Here's how the part is built. I have some questions about the finished solid (model axes, mm). Round coordinates to 2 decimals unless told otherwise and drop trailing zeros. Order: outer loops, then holes, each group sorted by start corner. A loop starts at its lowest first (then second) coordinate and runs counter-clockwise, first axis right, second up.
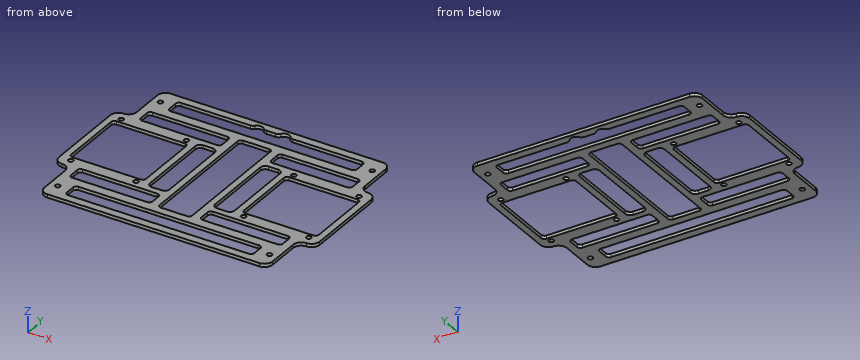
```python
from build123d import *

# Parameters (mm, degrees)
SKETCH_1_R          = 1.5
EXTRUDE_1_DEPTH     = 2
SKETCH_2_R          = 1.5
SKETCH_2_W          = 46
SKETCH_2_H          = 43
CUT_EXTRUDE_1_DEPTH = 2
FILLET_1_R          = 2
SKETCH_3_W          = 115
SKETCH_3_H          = 10
CUT_EXTRUDE_2_DEPTH = 2
FILLET_2_R          = 2
SKETCH_4_W          = 20
SKETCH_4_H          = 80
SKETCH_4_W_2        = 50
SKETCH_4_H_2        = 10
CUT_EXTRUDE_3_DEPTH = 2
FILLET_3_R          = 2
FILLET_4_R          = 5
SKETCH_5_R          = 3.5
CUT_EXTRUDE_4_DEPTH = 2
SKETCH_6_W          = 12
SKETCH_6_H          = 50
CUT_EXTRUDE_5_DEPTH = 2
FILLET_5_R          = 3


with BuildPart() as part:
    # 草图1 → 凸台-拉伸1 (new body)
    with BuildSketch(Plane.XY):
        Polygon((-70, -60), (70, -60), (70, -30), (80, -30), (80, 30), (70, 30), (70, 60), (-70, 60), (-70, 30), (-80, 30), (-80, -30), (-70, -30), align=None)
        with Locations((-65, 50)):
            Circle(SKETCH_1_R, mode=Mode.SUBTRACT)
        with Locations((65, 50)):
            Circle(SKETCH_1_R, mode=Mode.SUBTRACT)
        with Locations((65, -50)):
            Circle(SKETCH_1_R, mode=Mode.SUBTRACT)
        with Locations((-65, -50)):
            Circle(SKETCH_1_R, mode=Mode.SUBTRACT)
    extrude(amount=EXTRUDE_1_DEPTH)

    # 草图2 → 切除-拉伸1 (cut)
    with BuildSketch(Plane.XY.offset(2)):
        with Locations((-73, 24.5)):
            Circle(SKETCH_2_R)
        with Locations((-33, 24.5)):
            Circle(SKETCH_2_R)
        with Locations((-73, -24.5)):
            Circle(SKETCH_2_R)
        with Locations((-33, -24.5)):
            Circle(SKETCH_2_R)
        with Locations((33, 24.5)):
            Circle(SKETCH_2_R)
        with Locations((73, 24.5)):
            Circle(SKETCH_2_R)
        with Locations((33, -24.5)):
            Circle(SKETCH_2_R)
        with Locations((73, -24.5)):
            Circle(SKETCH_2_R)
        with Locations((53, 0)):
            Rectangle(SKETCH_2_W, SKETCH_2_H)
        with Locations((-53, 0)):
            Rectangle(SKETCH_2_W, SKETCH_2_H)
    extrude(amount=-CUT_EXTRUDE_1_DEPTH, mode=Mode.SUBTRACT)

    # 圆角1
    fillet_1_edges = [part.edges().sort_by_distance(p)[0] for p in [
        (76, 21.5, 1),
        (76, -21.5, 1),
        (30, -21.5, 1),
        (30, 21.5, 1),
        (-30, 21.5, 1),
        (-30, -21.5, 1),
        (-76, -21.5, 1),
        (-76, 21.5, 1),
    ]]
    fillet(fillet_1_edges, radius=FILLET_1_R)

    # 草图3 → 切除-拉伸2 (cut)
    with BuildSketch(Plane.XY.offset(2)):
        with Locations((0, -50)):
            Rectangle(SKETCH_3_W, SKETCH_3_H)
        with Locations((0, 50)):
            Rectangle(SKETCH_3_W, SKETCH_3_H)
    extrude(amount=-CUT_EXTRUDE_2_DEPTH, mode=Mode.SUBTRACT)

    # 圆角2
    fillet_2_edges = [part.edges().sort_by_distance(p)[0] for p in [
        (57.5, -45, 1),
        (57.5, -55, 1),
        (-57.5, -55, 1),
        (-57.5, -45, 1),
        (-57.5, 45, 1),
        (-57.5, 55, 1),
        (57.5, 55, 1),
        (57.5, 45, 1),
    ]]
    fillet(fillet_2_edges, radius=FILLET_2_R)

    # 草图4 → 切除-拉伸3 (cut)
    with BuildSketch(Plane.XY.offset(2)):
        Rectangle(SKETCH_4_W, SKETCH_4_H)
        with Locations((40, 34)):
            Rectangle(SKETCH_4_W_2, SKETCH_4_H_2)
        with Locations((-40, 34)):
            Rectangle(SKETCH_4_W_2, SKETCH_4_H_2)
        with Locations((40, -34)):
            Rectangle(SKETCH_4_W_2, SKETCH_4_H_2)
        with Locations((-40, -34)):
            Rectangle(SKETCH_4_W_2, SKETCH_4_H_2)
    extrude(amount=-CUT_EXTRUDE_3_DEPTH, mode=Mode.SUBTRACT)

    # 圆角3
    fillet_3_edges = [part.edges().sort_by_distance(p)[0] for p in [
        (-15, -29, 1),
        (-15, -39, 1),
        (-65, -39, 1),
        (-65, -29, 1),
        (15, -29, 1),
        (65, -29, 1),
        (65, -39, 1),
        (15, -39, 1),
        (-15, 39, 1),
        (-15, 29, 1),
        (-65, 29, 1),
        (-65, 39, 1),
        (65, 39, 1),
        (65, 29, 1),
        (15, 29, 1),
        (15, 39, 1),
        (10, 40, 1),
        (10, -40, 1),
        (-10, -40, 1),
        (-10, 40, 1),
    ]]
    fillet(fillet_3_edges, radius=FILLET_3_R)

    # 圆角4
    fillet_4_edges = [part.edges().sort_by_distance(p)[0] for p in [
        (70, -60, 1),
        (-70, -60, 1),
        (70, 30, 1),
        (80, 30, 1),
        (80, -30, 1),
        (70, -30, 1),
        (-70, -30, 1),
        (-80, -30, 1),
        (-80, 30, 1),
        (-70, 30, 1),
        (70, 60, 1),
        (-70, 60, 1),
    ]]
    fillet(fillet_4_edges, radius=FILLET_4_R - 0.0001)  # a hair under: the kernel refuses the full size

    # 草图5 → 切除-拉伸4 (cut)
    with BuildSketch(Plane.XY.offset(2)):
        with Locations((-8.036845279, 53.77878744)):
            Circle(SKETCH_5_R)
        with Locations((7.953054881, 54.34720003)):
            Circle(SKETCH_5_R)
    extrude(amount=-CUT_EXTRUDE_4_DEPTH, mode=Mode.SUBTRACT)

    # 草图6 → 切除-拉伸5 (cut)
    with BuildSketch(Plane.XY.offset(2)):
        with Locations((20, 0)):
            Rectangle(SKETCH_6_W, SKETCH_6_H)
        with Locations((-20, 0)):
            Rectangle(SKETCH_6_W, SKETCH_6_H)
    extrude(amount=-CUT_EXTRUDE_5_DEPTH, mode=Mode.SUBTRACT)

    # 圆角5
    fillet_5_edges = [part.edges().sort_by_distance(p)[0] for p in [
        (11.391637758, 55, 1),
        (4.514472005, 55, 1),
        (-4.756808711, 55, 1),
        (-11.316881846, 55, 1),
        (26, 25, 1),
        (26, -25, 1),
        (14, -25, 1),
        (14, 25, 1),
        (-14, 25, 1),
        (-14, -25, 1),
        (-26, -25, 1),
        (-26, 25, 1),
    ]]
    fillet(fillet_5_edges, radius=FILLET_5_R)


solid = part.part
```
1. I need wall thicknesses on probe 1 along Y at (x, z) = (-12.5, 0.5); probe 2 along X at (y, z) = (-19, 1.9); probe 3 along Y at (x, z) = (-28.5, 1.3). Which ranges of each line are inside material? Lowest first, please.
Evaluation:
probe 1: y = -60 to -55, -45 to 45, 55.04 to 60
probe 2: x = -80 to -76, -30 to -26, -14 to -10, 10 to 14, 26 to 30, 76 to 80
probe 3: y = -60 to -55, -45 to -39, -29 to 29, 39 to 45, 55 to 60
2. If we section it at A-A, the plane x = -37: Write out the boundary of the cut face in (y, z).
Evaluation:
outline: (-60, 0) - (-55, 0) - (-55, 2) - (-60, 2) - close; (-45, 0) - (-39, 0) - (-39, 2) - (-45, 2) - close; (-29, 0) - (-21.5, 0) - (-21.5, 2) - (-29, 2) - close; (21.5, 0) - (29, 0) - (29, 2) - (21.5, 2) - close; (39, 0) - (45, 0) - (45, 2) - (39, 2) - close; (55, 0) - (60, 0) - (60, 2) - (55, 2) - close
3. If we section it at B-B, the plane y = -13.5: Write out the boundary of the cut face in (x, z), and give its area (3 significant figures).
Evaluation:
outline: (-80, 0) - (-76, 0) - (-76, 2) - (-80, 2) - close; (-30, 0) - (-26, 0) - (-26, 2) - (-30, 2) - close; (-14, 0) - (-10, 0) - (-10, 2) - (-14, 2) - close; (10, 0) - (14, 0) - (14, 2) - (10, 2) - close; (26, 0) - (30, 0) - (30, 2) - (26, 2) - close; (76, 0) - (80, 0) - (80, 2) - (76, 2) - close
area: 48.0 mm2
4. If we section it at C-C, the plane z = 0.9: State how many separate pieces and enclosed holes the cut face has, and give its area (3 significant figures).
Evaluation:
separate pieces: 1
enclosed holes: 23
area: 6,860 mm2
5. I'm going to push flat-ended pins straight in: P1, Ø5, axis at x = -50, y = 32.5, coming from the +Z side (3 decimals); P2, Ø1, axis at y = -34, z = 1.5, coming from the +X side; P3, Ø0.6, axis at y = 51.5, z = 1, coming from the -X side. Where does each tip first touch, or does it pass through?
Evaluation:
P1: passes through
P2: stops at x = 70.23
P3: stops at x = -70
